Source: CAD feature listing. Evaluate the final solid. Frame: model axes, mm. A direction names the side the tool comes from. Give positions to 0.01 mm unless a question says otherwise; leave off trailing zeros. Loops run counter-clockwise (first coordinate to the right, second up) from the corner with the lowest first, then second, coordinate; pieces in that order, holes last. Notation, with made-up numbers: M 29.25,-29 L 57.25,-29 A24 cw 57.25,-10 Z; hole C 29,-14.75 d6. An arc over 180 degrees is marked long. Put each result on its own line as item: value. Start each with the question number.
```python
from build123d import *

# Parameters (mm, degrees)
SKETCH_1_R          = 8.5
EXTRUDE_1_DEPTH     = 2.5
SKETCH_2_R          = 9.5
EXTRUDE_2_DEPTH     = 2.5
EXTRUDE_3_DEPTH     = 28
SKETCH_4_W          = 26
SKETCH_4_H          = 26
EXTRUDE_5_DEPTH     = 2
EXTRUDE_6_DEPTH     = 2
SKETCH_7_R          = 1.1
CUT_EXTRUDE_1_DEPTH = 54.4976635


with BuildPart() as part:
    # ｽｹｯﾁ1 → ﾎﾞｽ - 押し出し1 (new body)
    with BuildSketch(Plane.XY):
        Circle(SKETCH_1_R)
    extrude(amount=EXTRUDE_1_DEPTH)

    # ｽｹｯﾁ2 → ﾎﾞｽ - 押し出し2 (add)
    with BuildSketch(Plane.XY.offset(2.5)):
        Circle(SKETCH_2_R)
    extrude(amount=EXTRUDE_2_DEPTH)

    # ｽｹｯﾁ3 → ﾎﾞｽ - 押し出し3 (add)
    with BuildSketch(Plane.XY.offset(5)):
        with BuildLine():
            Line((-26, 15.5), (2.5, 15.5))
            ThreePointArc((2.5, 15.5), (9.5, 0), (2.5, -15.5))
            Line((2.5, -15.5), (-26, -15.5))
            Line((-26, -15.5), (-26, -13))
            Line((-26, -13), (0, -13))
            Line((0, -13), (0, 13))
            Line((0, 13), (-26, 13))
            Line((-26, 13), (-26, 15.5))
        make_face()
    extrude(amount=EXTRUDE_3_DEPTH)

    # ｽｹｯﾁ4 → ﾎﾞｽ - 押し出し5 (add)
    with BuildSketch(Plane(origin=(0, 0, 5), x_dir=(-1, 0, 0), z_dir=(0, 0, -1))):
        with Locations((13, 0)):
            Rectangle(SKETCH_4_W, SKETCH_4_H)
    extrude(amount=-EXTRUDE_5_DEPTH)

    # ｽｹｯﾁ6 → ﾎﾞｽ - 押し出し6 (add)
    with BuildSketch(Plane.XY.offset(33)):
        with BuildLine():
            Line((-26, 15.5), (-26, -15.5))
            Line((-26, -15.5), (2.5, -15.5))
            ThreePointArc((2.5, -15.5), (9.5, 0), (2.5, 15.5))
            Line((2.5, 15.5), (-26, 15.5))
        make_face()
    extrude(amount=EXTRUDE_6_DEPTH)

    # ｽｹｯﾁ7 → ｶｯﾄ - 押し出し1 (cut, through all)
    with BuildSketch(Plane(origin=(0, 15.5, 0), x_dir=(1, 0, 0), z_dir=(0, 1, 0))):
        with Locations(Location((-23.5, -9.5, 0), (0, 0, 180))):
            Circle(SKETCH_7_R)
        with Locations(Location((-2.5, -9.5, 0), (0, 0, 180))):
            Circle(SKETCH_7_R)
        with Locations(Location((-2.5, -30.5, 0), (0, 0, 180))):
            Circle(SKETCH_7_R)
        with Locations(Location((-23.5, -30.5, 0), (0, 0, 180))):
            Circle(SKETCH_7_R)
    extrude(amount=-CUT_EXTRUDE_1_DEPTH, mode=Mode.SUBTRACT)


solid = part.part
```
1. Ray query, line 1 (Z direction, x = -23.5, y = -14.3); line 2 (Z direction, x = -12, y = 5.5); line 3 (Y direction, x = -21, z = 14.5). Return the intervals inside material, ascending.
2. Section D-D, the plane z = 17. Output: boundary loops of the cut face in (x, y).
3. Contact query for flat-ended pins moving along their axis: pin 1 (2.5 mm diameter, centred on x = -23.5, z = 30.5, fed in from -Y); pin 2 (8 mm diameter, centred on y = -3.5, z = 18, fed in from -X); pin 3 (13 mm diameter, centred on x = -19, y = 0.5, fed in from -Z). Output: stop coordinate, or through.
4. Section A-A, the plane z = 30.5. Output: boundary loops of the cut face in (x, y).
5. Set-up query: faces 1 (the face through (0, 0, 20)), 2 (the face through (4.38, -8.43, 3.73)), 3 (the face through (-3.008, -14.233, 29.524)). Return all of +Z, -Z, +X, -X, +Y, -Y with unobstructed straight access to the full face (end or side cutting, diameter ignored); none if empty.
6. Section C-C, the plane y = 13.5. Output: boundary loops of the cut face in (x, z), plus the area to 3 significant figures.
7. Pull-direction query (X, two-part tool) for faces 4 (the face through (4.57, 7.167, 1.232)), 5 (the face through (-12, 15.5, 20)), 6 (the face through (-3.516, -14.233, 9.079)), 7 (the face through (9.5, -0.2, 19.8)); classes: released by +X, released by -X, zero draft, split by the parting line, or undercut.
8. Section B-B, the plane x = -23.5. Output: boundary loops of the cut face in (y, z), plus the area to 3 significant figures.
Results found:
1. line 1: 5 to 8.4, 10.6 to 29.4, 31.6 to 35
1. line 2: 5 to 7, 33 to 35
1. line 3: -15.5 to -13, 13 to 15.5
2. outline: M -26,-15.5 L 2.5,-15.5 A20.66 ccw 2.5,15.5 L -26,15.5 L -26,13 L 0,13 L 0,-13 L -26,-13 Z
3. pin 1: y = -15.5
3. pin 2: x = 0
3. pin 3: z = 5
4. outline: M -26,-15.5 L -24.6,-15.5 L -24.6,-13 L -26,-13 Z; M -26,13 L -24.6,13 L -24.6,15.5 L -26,15.5 Z; M -22.4,-15.5 L -3.6,-15.5 L -3.6,-13 L -22.4,-13 Z; M -22.4,13 L -3.6,13 L -3.6,15.5 L -22.4,15.5 Z; M -1.4,-15.5 L 2.5,-15.5 A20.66 ccw 2.5,15.5 L -1.4,15.5 L -1.4,13 L 0,13 L 0,-13 L -1.4,-13 Z
5. face 1: -X
5. face 2: -Z
5. face 3: +Y, -Y
6. outline: M -26,5 L 4.48,5 L 4.48,35 L -26,35 Z; hole C -23.5,9.5 d2.2; hole C -23.5,30.5 d2.2; hole C -2.5,9.5 d2.2; hole C -2.5,30.5 d2.2
6. area: 899 mm²
7. face 4: split by the parting line
7. face 5: zero draft
7. face 6: undercut
7. face 7: released by +X
8. outline: M -15.5,5 L 15.5,5 L 15.5,8.4 L 13,8.4 L 13,7 L -13,7 L -13,8.4 L -15.5,8.4 Z; M -15.5,10.6 L -13,10.6 L -13,29.4 L -15.5,29.4 Z; M -15.5,31.6 L -13,31.6 L -13,33 L 13,33 L 13,31.6 L 15.5,31.6 L 15.5,35 L -15.5,35 Z; M 13,10.6 L 15.5,10.6 L 15.5,29.4 L 13,29.4 Z
8. area: 232 mm²
